Here's how the part is built. I have some questions about the finished solid (model axes, mm). A direction names the side the tool comes from. Give positions to 0.01 mm unless a question says otherwise; leave off trailing zeros. Order: outer loops, then holes, each group sorted by start corner. A loop starts at its lowest first (then second) coordinate and runs counter-clockwise, first axis right, second up. Notation, with made-up numbers: (75.5, -31.75) - (96.5, -31.75) arc R5 ccw to (96.5, -25.75) - close; hole circle Ø1 at (-30.75, 62). An arc over 180 degrees is marked (long way). One line per question, with ' | ' between items.
from build123d import *

# Parameters (mm, degrees)
SKETCH_W          = 43
SKETCH_H          = 24
SKETCH_R          = 1.6
PAD_DEPTH         = 2
SKETCH001_W       = 19
SKETCH001_H       = 38
PAD001_DEPTH      = 2
SKETCH002_R       = 1.6
PAD002_DEPTH      = 2
SKETCH005_R       = 1.6
PAD003_DEPTH      = 2
SKETCH004_R       = 1.6
POCKET_DEPTH      = 21.501
POCKET_DEPTH_BACK = -21.501
FILLET_R          = 2
FILLET001_R       = 8.99
CHAMFER_SIZE      = 4
CHAMFER001_SIZE   = 13
FILLET002_R       = 13
FILLET003_R       = 3


with BuildPart() as part:
    # Sketch → Pad (new body)
    with BuildSketch(Plane.XZ):
        with Locations((0, 12)):
            Rectangle(SKETCH_W, SKETCH_H)
        with Locations((-19, 21)):
            Circle(SKETCH_R, mode=Mode.SUBTRACT)
        with Locations((-19, 11)):
            Circle(SKETCH_R, mode=Mode.SUBTRACT)
        with Locations((19, 11)):
            Circle(SKETCH_R, mode=Mode.SUBTRACT)
        with Locations((19, 21)):
            Circle(SKETCH_R, mode=Mode.SUBTRACT)
    extrude(amount=PAD_DEPTH)

    # Sketch001 → Pad001 (join)
    with BuildSketch(Plane.XY):
        with Locations((0, -19)):
            Rectangle(SKETCH001_W, SKETCH001_H)
        Polygon((7.5, -17), (7.5, -36), (-7.5, -36), (-7.5, -17), (0, -17), (0, -15.5), (2, -15.5), (2, -17), align=None, mode=Mode.SUBTRACT)
    extrude(amount=PAD001_DEPTH)

    # Sketch002 (on DatumPlane) → Pad002 (join)
    with BuildSketch(Plane.YZ.offset(-9.5)):
        Polygon((0, 24), (0, 0), (-38, 0), (-38, 12), (-29, 12), (-29, 48), (-17, 48), (-17, 24), align=None)
        with Locations((-21, 44)):
            Circle(SKETCH002_R, mode=Mode.SUBTRACT)
    extrude(amount=PAD002_DEPTH)

    # Sketch005 (on DatumPlane) → Pad003 (join)
    with BuildSketch(Plane.YZ.offset(9.5)):
        Polygon((0, 24), (0, 0), (-38, 0), (-38, 12), (-29, 12), (-29, 48), (-17, 48), (-17, 24), align=None)
        with Locations((-21, 44)):
            Circle(SKETCH005_R, mode=Mode.SUBTRACT)
    extrude(amount=-PAD003_DEPTH)

    # Sketch004 → Pocket (cut, two sides)
    with BuildSketch(Plane.YZ) as pocket_sk:
        with Locations((-15, 15)):
            Circle(SKETCH004_R)
    extrude(amount=-POCKET_DEPTH, mode=Mode.SUBTRACT)
    extrude(pocket_sk.sketch, amount=-POCKET_DEPTH_BACK, mode=Mode.SUBTRACT)

    # Fillet
    fillet_edges = [part.edges().sort_by_distance(p)[0] for p in [
        (9.5, -2, 13),
        (-9.5, -2, 13),
    ]]
    fillet(fillet_edges, radius=FILLET_R)

    # Fillet001
    fillet001_edges = [part.edges().sort_by_distance(p)[0] for p in [
        (8.5, -29, 12),
        (-8.5, -29, 12),
    ]]
    fillet(fillet001_edges, radius=FILLET001_R)

    # Chamfer
    chamfer_edges = [part.edges().sort_by_distance(p)[0] for p in [
        (8.5, -38, 12),
        (-8.5, -38, 12),
    ]]
    chamfer(chamfer_edges, length=CHAMFER_SIZE)

    # Chamfer001
    chamfer001_edges = [part.edges().sort_by_distance(p)[0] for p in [
        (0, -2, 2),
    ]]
    chamfer(chamfer001_edges, length=CHAMFER001_SIZE)

    # Fillet002
    fillet002_edges = [part.edges().sort_by_distance(p)[0] for p in [
        (8.5, -17, 24),
        (-8.5, -17, 24),
    ]]
    fillet(fillet002_edges, radius=FILLET002_R)

    # Fillet003
    fillet003_edges = [part.edges().sort_by_distance(p)[0] for p in [
        (8.5, -29, 48),
        (-8.5, -29, 48),
        (-8.5, -17, 48),
        (8.5, -17, 48),
    ]]
    fillet(fillet003_edges, radius=FILLET003_R)


solid = part.part
1) On a 3-axis mill with a long thin cutter (end or side, diameter ignored), from which of +Z, -Z, +X, -X, +Y, -Y can I reach the whole of each face in a straight line? I mean faces 1 (the face through (-9, -29, 33)), 2 (the face through (0, -16, 1)), 3 (the face through (-9, -17, 41)), 4 (the face through (16, -2, 12)), 5 (the face through (0, -9, 8)). Say none if no direction works.
Model answer:
face 1: +Z, +X, -X, -Y | face 2: +Z, -Z | face 3: +Z, +X, -X, +Y | face 4: +Z, -Z, +X, -Y | face 5: +Z, -Y
2) Please list where these lines run through material, in increasing order: L1, parallel to Z at x = 19, y = -0.65; L2, parallel to Z at x = -8.05, y = -21; L3, parallel to X at y = -20, z = 27.
Model answer:
L1: z = 0 to 9.4, 12.6 to 19.4, 22.6 to 24 | L2: z = 0 to 42.4, 45.6 to 48 | L3: x = -9.5 to -7.5, 7.5 to 9.5
3) I want a section at D-D (x = 19). List the corners of the cut face in (y, z) for me.
Model answer:
outline: (-2, 0) - (0, 0) - (0, 9.4) - (-2, 9.4) - close; (-2, 12.6) - (0, 12.6) - (0, 19.4) - (-2, 19.4) - close; (-2, 22.6) - (0, 22.6) - (0, 24) - (-2, 24) - close
4) I want a section at B-B (z = 44). List the corners of the cut face in (x, y) for me, plus the area to 3 significant figures.
Model answer:
outline: (-9.5, -29) - (-7.5, -29) - (-7.5, -22.6) - (-9.5, -22.6) - close; (-9.5, -19.4) - (-7.5, -19.4) - (-7.5, -17) - (-9.5, -17) - close; (7.5, -29) - (9.5, -29) - (9.5, -22.6) - (7.5, -22.6) - close; (7.5, -19.4) - (9.5, -19.4) - (9.5, -17) - (7.5, -17) - close | area: 35.2 mm2
5) I'm going to push flat-ended pins straight in: P1, Ø2, axis at x = -8, z = 36, coming from the -Y side; P2, Ø8, axis at x = -16, z = 12, coming from the -Y side; P3, Ø5, axis at x = 0, z = 8.5, coming from the -Y side. Where does each tip first touch, or does it pass through?
Model answer:
P1: stops at y = -29 | P2: stops at y = -2 | P3: stops at y = -11
6) Thinking about a two-plate mould opening in Z: for faces 6 (the face through (-8.486, -13.091, 27.707)), 7 (the face through (17.82, -0.99, 12.08)), 8 (the face through (0, -38, 1)), which applies, +Z half, -Z half, draft (parallel to the pull), parting line (faces both ways), or undercut?
Model answer:
face 6: +Z half | face 7: undercut | face 8: draft
7) I want a section at C-C (y = -24). List the corners of the cut face in (x, z) for me, plus the area to 3 significant figures.
Model answer:
outline: (-9.5, 0) - (-7.5, 0) - (-7.5, 48) - (-9.5, 48) - close; (7.5, 0) - (9.5, 0) - (9.5, 48) - (7.5, 48) - close | area: 192 mm2
8) I want a section at A-A (x = 4.5). List the corners of the cut face in (y, z) for me, plus the area to 4 significant figures.
Model answer:
outline: (-38, 0) - (-36, 0) - (-36, 2) - (-38, 2) - close; (-17, 0) - (0, 0) - (0, 24) - (-2, 24) - (-2, 15) - (-15, 2) - (-17, 2) - close | area: 166.5 mm2
